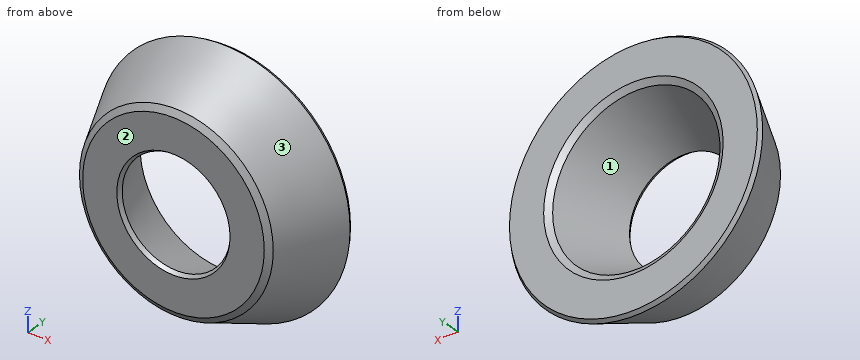
Autodesk Inventor part; units mm, degrees
ref_plane "YZ Plane" through (0, 0, 0) normal (1, 0, 0) x (0, 1, 0)
ref_plane "XZ Plane" through (0, 0, 0) normal (0, 1, 0) x (-1, 0, 0)
ref_plane "XY Plane" through (0, 0, 0) normal (0, 0, 1) x (1, 0, 0)
sketch "Sketch1" plane through (0, 0, 0) normal (0, 0, 1) x (1, 0, 0)
  line L0 (0, 0) -> (0, 3.3)
  line L1 (2.45, 0) -> (4.45, 0)
  line L2 (4.45, 0) -> (6, 3.3)
  line L3 (6, 3.3) -> (4, 3.3)
  line L4 (4, 3.3) -> (2.45, 0)
  point P0 (3.45, 0)
  point P1 (5, 3.3)
  dimension "d1" = 3.3
  dimension "d3" = 2
  dimension "d5" = 8
  dimension "d6" = 4.9
revolve "Revolution1" add sketch "Sketch1" angle 360 about axis through (0, 0, 0) along (0, 1, 0)
chamfer "Chamfer1" distance 0.2 angle 45 4 edges at (-6, 3.3, 0) (-4.45, 0, 0) (-4, 3.3, 0) (-2.45, 0, 0)
properties part number "Washer"
Build history of the part. All positions in model axes, mm. Face numbers are marked on the shaded views. Round coordinates to 2 decimals unless told otherwise and drop trailing zeros. Loops run counter-clockwise (first coordinate to the right, second up) from the corner with the lowest first, then second, coordinate; pieces in that order, holes last. Notation, with made-up numbers: (-31.5, -39) -> (-15.5, -39) arc R18 cw to (-15.5, -26) -> close; hole circle Ø9 at (75, -13.5). An arc over 180 degrees is marked (long way). Answer in a Markdown table with one row per item.
Item 1: Saw through at D-D (y = 1.75). Write the cut outline in (x, z), and give its area (3 significant figures).
Answers below:
| item | result |
|---|---|
| outline | circle Ø10.54 at (0, 0); hole circle Ø6.54 at (0, 0) |
| area | 53.7 mm² |
Item 2: Saw through at A-A (x = 0). Write the cut outline in (y, z).
Answers below:
| item | result |
|---|---|
| outline | (0, -4.25) -> (0.18, -4.54) -> (3.12, -5.91) -> (3.3, -5.8) -> (3.3, -4.2) -> (3.12, -3.91) -> (0.18, -2.54) -> (0, -2.65) -> close; (0, 2.65) -> (0.18, 2.54) -> (3.12, 3.91) -> (3.3, 4.2) -> (3.3, 5.8) -> (3.12, 5.91) -> (0.18, 4.54) -> (0, 4.25) -> close |
Item 3: Saw through at C-C (y = 2.75). Write the cut outline in (x, z), and give its area (3 significant figures).
Answers below:
| item | result |
|---|---|
| outline | circle Ø11.48 at (0, 0); hole circle Ø7.48 at (0, 0) |
| area | 59.6 mm² |
Item 4: Saw through at B-B (z = 0). Write the cut outline in (x, y), and give its area (3 significant figures).
Answers below:
| item | result |
|---|---|
| outline | (-5.91, 3.12) -> (-4.54, 0.18) -> (-4.25, 0) -> (-2.65, 0) -> (-2.54, 0.18) -> (-3.91, 3.12) -> (-4.2, 3.3) -> (-5.8, 3.3) -> close; (2.54, 0.18) -> (2.65, 0) -> (4.25, 0) -> (4.54, 0.18) -> (5.91, 3.12) -> (5.8, 3.3) -> (4.2, 3.3) -> (3.91, 3.12) -> close |
| area | 13.1 mm² |
Item 5: Mould opens along Z. For the marked faces 1, 2 and 3 say: +Z half, -Z half, draft (parallel to the pull), parting line (faces both ways), or undercut.
Answers below:
| item | result |
|---|---|
| face 1 | undercut |
| face 2 | draft |
| face 3 | parting line |
Item 6: Drill centre lines: L1, parallel to Z at x = 3, y = 2.4; L2, parallel to X at y = 2.15, z = 0.25; L3, parallel to Z at x = 2.5, y = 2.25. Where is each one in solid material? Low to high. Write a range as [from, to].
Answers below:
| item | result |
|---|---|
| L1 | z = [-4.7, -1.95], [1.95, 4.7] |
| L2 | x = [-5.45, -3.45], [3.45, 5.45] |
| L3 | z = [-4.91, -2.46], [2.46, 4.91] |
